from build123d import *

# Parameters (mm, degrees)
SZKIC1_R                    = 30
DODANIE_WYCI_GNI_CIE1_DEPTH = 30


with BuildPart() as part:
    # Szkic1 → Dodanie-wyciągnięcie1 (new body)
    with BuildSketch(Plane.XY):
        with BuildLine():
            Line((-48.200266446, 55.220649807), (-47.516798881, 60.795035566))
            Line((-47.516798881, 60.795035566), (-44.510409747, 67.354430039))
            ThreePointArc((-44.510409747, 67.354430039), (-43.078000693, 68.471781184), (-41.280473034, 68.734770905))
            Line((-41.280473034, 68.734770905), (-36.499658689, 68.734770905))
            ThreePointArc((-36.499658689, 68.734770905), (-34.70213103, 68.471781184), (-33.269721976, 67.354430039))
            Line((-33.269721976, 67.354430039), (-30.263332842, 60.795035566))
            Line((-30.263332842, 60.795035566), (-29.579865278, 55.220649807))
            ThreePointArc((-29.579865278, 55.220649807), (-21.585114177, 53.259164913), (-13.964292777, 50.146842733))
            Line((-13.964292777, 50.146842733), (-10.134814162, 54.254883391))
            Line((-10.134814162, 54.254883391), (-3.847078926, 57.794433797))
            ThreePointArc((-3.847078926, 57.794433797), (-2.031473134, 57.856440945), (-0.42266123, 57.01264385))
            Line((-0.42266123, 57.01264385), (3.445098822, 54.202551684))
            ThreePointArc((3.445098822, 54.202551684), (4.744747767, 52.933228281), (5.24682851, 51.187323299))
            Line((5.24682851, 51.187323299), (3.823533075, 44.113550502))
            Line((3.823533075, 44.113550502), (1.09992821, 39.202045535))
            ThreePointArc((1.09992821, 39.202045535), (6.414885823, 32.915974128), (10.75088277, 25.918646164))
            Line((10.75088277, 25.918646164), (16.263641763, 26.991209816))
            Line((16.263641763, 26.991209816), (23.431021953, 26.158928205))
            ThreePointArc((23.431021953, 26.158928205), (24.936324781, 25.141906732), (25.741909464, 23.513624632))
            Line((25.741909464, 23.513624632), (27.219262344, 18.966799996))
            ThreePointArc((27.219262344, 18.966799996), (27.52461085, 17.17598131), (26.904585503, 15.468398852))
            Line((26.904585503, 15.468398852), (21.595255981, 10.582188511))
            Line((21.595255981, 10.582188511), (16.504903173, 8.209592297))
            ThreePointArc((16.504903173, 8.209592297), (17.109934138, 0), (16.504903173, -8.209592297))
            Line((16.504903173, -8.209592297), (21.595255981, -10.582188511))
            Line((21.595255981, -10.582188511), (26.904585503, -15.468398852))
            ThreePointArc((26.904585503, -15.468398852), (27.52461085, -17.17598131), (27.219262344, -18.966799996))
            Line((27.219262344, -18.966799996), (25.741909464, -23.513624632))
            ThreePointArc((25.741909464, -23.513624632), (24.936324781, -25.141906732), (23.431021953, -26.158928205))
            Line((23.431021953, -26.158928205), (16.263641763, -26.991209816))
            Line((16.263641763, -26.991209816), (10.75088277, -25.918646164))
            ThreePointArc((10.75088277, -25.918646164), (6.414885823, -32.915974128), (1.09992821, -39.202045535))
            Line((1.09992821, -39.202045535), (3.823533075, -44.113550502))
            Line((3.823533075, -44.113550502), (5.24682851, -51.187323299))
            ThreePointArc((5.24682851, -51.187323299), (4.744747767, -52.933228281), (3.445098822, -54.202551684))
            Line((3.445098822, -54.202551684), (-0.42266123, -57.01264385))
            ThreePointArc((-0.42266123, -57.01264385), (-2.031473134, -57.856440945), (-3.847078926, -57.794433797))
            Line((-3.847078926, -57.794433797), (-10.134814162, -54.254883391))
            Line((-10.134814162, -54.254883391), (-13.964292777, -50.146842733))
            ThreePointArc((-13.964292777, -50.146842733), (-21.585114177, -53.259164913), (-29.579865278, -55.220649807))
            Line((-29.579865278, -55.220649807), (-30.263332842, -60.795035566))
            Line((-30.263332842, -60.795035566), (-33.269721976, -67.354430039))
            ThreePointArc((-33.269721976, -67.354430039), (-34.70213103, -68.471781184), (-36.499658689, -68.734770905))
            Line((-36.499658689, -68.734770905), (-41.280473034, -68.734770905))
            ThreePointArc((-41.280473034, -68.734770905), (-43.078000693, -68.471781184), (-44.510409747, -67.354430039))
            Line((-44.510409747, -67.354430039), (-47.516798881, -60.795035566))
            Line((-47.516798881, -60.795035566), (-48.200266446, -55.220649807))
            ThreePointArc((-48.200266446, -55.220649807), (-56.195017547, -53.259164913), (-63.815838947, -50.146842733))
            Line((-63.815838947, -50.146842733), (-67.645317562, -54.254883391))
            Line((-67.645317562, -54.254883391), (-73.933052797, -57.794433797))
            ThreePointArc((-73.933052797, -57.794433797), (-75.74865859, -57.856440945), (-77.357470494, -57.01264385))
            Line((-77.357470494, -57.01264385), (-81.225230545, -54.202551684))
            ThreePointArc((-81.225230545, -54.202551684), (-82.52487949, -52.933228281), (-83.026960233, -51.187323299))
            Line((-83.026960233, -51.187323299), (-81.603664799, -44.113550502))
            Line((-81.603664799, -44.113550502), (-78.880059934, -39.202045535))
            ThreePointArc((-78.880059934, -39.202045535), (-84.195017547, -32.915974128), (-88.531014493, -25.918646164))
            Line((-88.531014493, -25.918646164), (-94.043773486, -26.991209816))
            Line((-94.043773486, -26.991209816), (-101.211153677, -26.158928205))
            ThreePointArc((-101.211153677, -26.158928205), (-102.716456505, -25.141906732), (-103.522041188, -23.513624632))
            Line((-103.522041188, -23.513624632), (-104.999394067, -18.966799996))
            ThreePointArc((-104.999394067, -18.966799996), (-105.304742573, -17.17598131), (-104.684717227, -15.468398852))
            Line((-104.684717227, -15.468398852), (-99.375387704, -10.582188511))
            Line((-99.375387704, -10.582188511), (-94.285034896, -8.209592297))
            ThreePointArc((-94.285034896, -8.209592297), (-94.890065862, 0), (-94.285034896, 8.209592297))
            Line((-94.285034896, 8.209592297), (-99.375387704, 10.582188511))
            Line((-99.375387704, 10.582188511), (-104.684717227, 15.468398852))
            ThreePointArc((-104.684717227, 15.468398852), (-105.304742573, 17.17598131), (-104.999394067, 18.966799996))
            Line((-104.999394067, 18.966799996), (-103.522041188, 23.513624632))
            ThreePointArc((-103.522041188, 23.513624632), (-102.716456505, 25.141906732), (-101.211153677, 26.158928205))
            Line((-101.211153677, 26.158928205), (-94.043773486, 26.991209816))
            Line((-94.043773486, 26.991209816), (-88.531014493, 25.918646164))
            ThreePointArc((-88.531014493, 25.918646164), (-84.195017547, 32.915974128), (-78.880059934, 39.202045535))
            Line((-78.880059934, 39.202045535), (-81.603664799, 44.113550502))
            Line((-81.603664799, 44.113550502), (-83.026960233, 51.187323299))
            ThreePointArc((-83.026960233, 51.187323299), (-82.52487949, 52.933228281), (-81.225230545, 54.202551684))
            Line((-81.225230545, 54.202551684), (-77.357470494, 57.01264385))
            ThreePointArc((-77.357470494, 57.01264385), (-75.74865859, 57.856440945), (-73.933052797, 57.794433797))
            Line((-73.933052797, 57.794433797), (-67.645317562, 54.254883391))
            Line((-67.645317562, 54.254883391), (-63.815838947, 50.146842733))
            ThreePointArc((-63.815838947, 50.146842733), (-56.195017547, 53.259164913), (-48.200266446, 55.220649807))
        make_face()
        with Locations((-38.890065862, 0)):
            Circle(SZKIC1_R, mode=Mode.SUBTRACT)
    extrude(amount=DODANIE_WYCI_GNI_CIE1_DEPTH)


solid = part.part
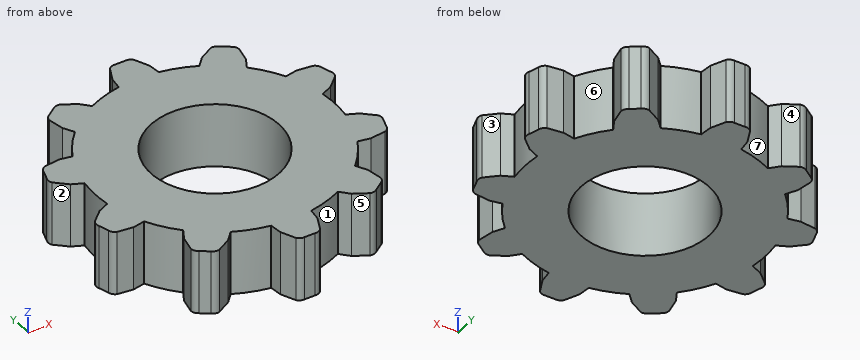
Verification items for the finished model (mm, model axes). Face numbers are marked on the shaded views. A direction names the side the tool comes from. Coordinates: 2 decimals unless noted, no trailing zeros. Order: outer loops, then holes, each group sorted by start corner. A loop starts at its lowest first (then second) coordinate and runs counter-clockwise, first axis right, second up.
Item 1: Release check for a two-part mould opening along Y. For the marked faces 5, 6 and 7 record: +Y half, -Y half, draft (parallel to the pull), parting line (faces both ways), or undercut.
Filled in:
face 5: -Y half
face 6: undercut
face 7: +Y half
Item 2: Section check A-A, the plane y = 0. Enter the section's corners in (x, z), then the cut area to 3 significant figures.
Filled in:
outline: (-94.89, 0) - (-68.89, 0) - (-68.89, 30) - (-94.89, 30) - close; (-8.89, 0) - (17.11, 0) - (17.11, 30) - (-8.89, 30) - close
area: 1,560 mm2
Item 3: Depth check by flat-ended pin: pin 1 (10 mm diameter, centred on y = 43, z = 3.5, fed in from -X); pin 2 (10 mm diameter, centred on x = -50, z = 25.5, fed in from +Y); pin 3 (8 mm diameter, centred on y = 3.5, z = 15, fed in from +X). Enter the tip coordinate at first touch or a pass-through.
Filled in:
pin 1: stops at x = -82.39
pin 2: stops at y = 66.29
pin 3: stops at x = 17.11
Item 4: Material ranges on L1, parallel to Y at x = 3.5, z = 25.75; L2, parallel to Y at x = -17, z = 27; L3, parallel to Y at x = -55, z = 22.5, recorded low to high.
Filled in:
L1: y = -54.17 to -43.53, -36.59 to 36.59, 43.53 to 54.17
L2: y = -51.54 to -20.51, 20.51 to 51.54
L3: y = -53.63 to -25.31, 25.31 to 53.63
Item 5: Section check B-B, the plane x = -17. Enter the section's corners in (y, z).
Filled in:
outline: (-51.54, 0) - (-20.51, 0) - (-20.51, 30) - (-51.54, 30) - close; (20.51, 0) - (51.54, 0) - (51.54, 30) - (20.51, 30) - close
Item 6: Access from +Z, -Z, +X, -X, +Y, -Y to the whole of each face (thin tool, end or side, straight path). Record for the marked faces 1, 2, 3 and 4.
Filled in:
face 1: +Z, -Z, -Y
face 2: +Z, -Z, -X
face 3: +Z, -Z, +X
face 4: +Z, -Z, +Y
Item 7: Section check C-C, the plane y = -36. Enter the section's corners in (x, z).
Filled in:
outline: (-81.79, 0) - (4.01, 0) - (4.01, 30) - (-81.79, 30) - close
